Autodesk Inventor part; units mm, degrees
ref_plane "YZ Plane" through (0, 0, 0) normal (1, 0, 0) x (0, 1, 0)
ref_plane "XZ Plane" through (0, 0, 0) normal (0, 1, 0) x (-1, 0, 0)
ref_plane "XY Plane" through (0, 0, 0) normal (0, 0, 1) x (1, 0, 0)
sketch "Sketch1" plane through (0, 0, 0) normal (0, 1, 0) x (-1, 0, 0)
  line L0 (0, 0) -> (0, 33)
  line L1 (0, 33) -> (5, 33)
  line L2 (0, 0) -> (0, 11) construction
  line L3 (0, 11) -> (0, 22) construction
  line L4 (0, 22) -> (0, 33) construction
  line L5 (0, 22) -> (5, 22) construction
  line L6 (0, 11) -> (5, 11) construction
  line L7 (5, 33) -> (2.5, 22)
  line L8 (2.5, 22) -> (5, 22)
  line L9 (5, 22) -> (2.5, 11)
  line L10 (4.8494, 11) -> (2.5, 11)
  line L11 (0, 0) -> (5, 0) construction
  line L12 (4.8494, 11) -> (2.5, 0)
  line L13 (0, 0) -> (2.5, 0)
  dimension "d0" = 33
  dimension "d1" = 5
  dimension "d13" = 11
  dimension "d14" = 11
  dimension "d15" = 5
  dimension "d16" = 5
  dimension "d17" = 5
extrude "Extrusion1" add sketch "Sketch1" along normal blind 1
fillet "Fillet1" radius 0.5 2 edges at (-2.5, 0.5, 11) (-2.5, 0.5, 22)
properties part number "spikyboi" material "Titanium"
For this review, take the finished solid that the model builds, in its own axes (mm). A direction names the side the tool comes from. Coordinates: 2 decimals unless noted, no trailing zeros. Write each loop counter-clockwise with the first axis right and the second up, starting at its lowest first coordinate (ties: lowest second). Pieces come first, ordered by that corner, then holes. Notation, with made-up numbers: (-15, -6) -> (35, -6) arc R20 ccw to (35, 16) -> close; hole circle Ø8 at (61.5, 46.5). An arc over 180 degrees is marked (long way). Write each question's results on one line, items separated by ' | '. Start each with the question number.
1) The part is to be moulded in two halves that separate along Z. For faces 3 (the face through (-1.2, 0.5, 0)), 4 (the face through (0, 0.5, 16.3)), 5 (the face through (-4, 0.5, 11)), 6 (the face through (-3.836, 0.493, 27.878)), say which applies: +Z half, -Z half, draft (parallel to the pull), parting line (faces both ways), or undercut.
2) Consider section A-A (x = -4.3). Write out the cut boundary in (y, z), plus the area to 3 significant figures.
3) Wall thickness on L1, parallel to X at y = 0.4, z = 15; L2, parallel to X at y = 0.4, z = 25: over which ranges is each line inside the solid? List them lowest first. Write a range as [from, to].
4) Consider section C-C (z = 27.5). Write out the cut boundary in (x, y).
5) For faces 1 (the face through (-3.836, 0.493, 16.878)), 2 (the face through (-3.69, 0.49, 5.58)), list the 3-axis set-ups (+Z, -Z, +X, -X, +Y, -Y) from which the entire face can be reached by the end or side of a thin tool; tool diameter is ignored.
6) Consider section D-D (z = 2.5). Write out the cut boundary in (x, y), plus the area to 3 significant figures.
7) Consider section B-B (y = 0.8). Write out the cut boundary in (x, z).
Geometry says:
1) face 3: -Z half | face 4: draft | face 5: undercut | face 6: undercut
2) outline: (0, 8.43) -> (1, 8.43) -> (1, 11) -> (0, 11) -> close; (0, 18.92) -> (1, 18.92) -> (1, 22) -> (0, 22) -> close; (0, 29.92) -> (1, 29.92) -> (1, 33) -> (0, 33) -> close | area: 8.73 mm^2
3) L1: [-3.41, 0] | L2: [-3.18, 0]
4) outline: (-3.75, 0) -> (0, 0) -> (0, 1) -> (-3.75, 1) -> close
5) face 1: -X, +Y, -Y | face 2: -Z, -X, +Y, -Y
6) outline: (-3.03, 0) -> (0, 0) -> (0, 1) -> (-3.03, 1) -> close | area: 3.03 mm^2
7) outline: (-5, 22) -> (-2.64, 11.61) arc R0.5 cw to (-3.13, 11) -> (-4.85, 11) -> (-2.5, 0) -> (0, 0) -> (0, 33) -> (-5, 33) -> (-2.64, 22.61) arc R0.5 cw to (-3.13, 22) -> close
